The model under review builds one solid part; all positions refer to its coordinate system, in mm. A direction names the side the tool comes from. Round coordinates to 2 decimals unless told otherwise and drop trailing zeros. Write each loop counter-clockwise with the first axis right and the second up, starting at its lowest first coordinate (ties: lowest second). Pieces come first, ordered by that corner, then holes. Notation, with made-up numbers: (65, 50) -> (84, 50) arc R22 cw to (84, 68) -> close; hole circle Ø5 at (-35, 16.25). An arc over 180 degrees is marked (long way). Return JSON: item names as keys, results as strings. Group by question number.
1. Take a section at D-D, the plane x = 2.5. Write out the cut boundary in (y, z), then the cut area to 3 significant figures.
2. Clearance check with flat-ended pins moving along their axes: P1, Ø4, axis at y = 3.5, z = -2.5, coming from the -X side; P2, Ø3, axis at x = -40, y = 3.5, coming from the -Z side; P3, Ø4, axis at x = -3.5, y = 2, coming from the +Z side. State where each tip first meets the part, or that it passes through.
3. Take a section at A-A, the plane z = -2.5. Write out the cut boundary in (x, y).
4. For line 1 along Y through (x, z) = (4.5, -2.5); line 2 along X through (y, z) = (3.5, 9.75); line 3 along X through (y, z) = (3.5, 12.75), list the stretches that pass through material, from the lowest coordinate up. Write a range as from..to.
5. Tool access review of faces 1 (the flat face through (-22, 3, 7.5)), 2 (the flat face through (7, 3, -18)), 3 (the flat face through (-27, 3, 14.5)), 4 (the flat face through (3, 3, -35)): name each direction out of +Z, -Z, +X, -X, +Y, -Y from which nothing blocks a thin tool from reaching the whole face with its end or side.
6. Take a section at B-B, the plane x = -10. Write out the cut boundary in (y, z), then the cut area to 3 significant figures.
7. Mouldability with a two-part tool opening along Z and no side actions: class faces 5 (the flat face through (2.59, 3.45, 20.65)), 6 (the cylindrical face through (-39.01, 2.74, 10.95)), 7 (the cylindrical face through (3.451, 3.021, -31.345)) as pulls with the +Z half, pulls with the -Z half, needs draft (parallel to the pull), parting line crosses it, or undercut.
8. Take a section at C-C, the plane y = 1. Write out the cut boundary in (x, z).
Autodesk Inventor part; units mm, degrees
ref_plane "YZ Plane" through (0, 0, 0) normal (1, 0, 0) x (0, 1, 0)
ref_plane "XZ Plane" through (0, 0, 0) normal (0, 1, 0) x (-1, 0, 0)
ref_plane "XY Plane" through (0, 0, 0) normal (0, 0, 1) x (1, 0, 0)
sketch "Sketch1" plane through (0, 0, 0) normal (0, 1, 0) x (-1, 0, 0)
  line L0 (0, 0) -> (16.4443, 0)
  line L1 (0, 0) -> (0, -35)
  line L2 (0, -17.5) -> (0, 7.5)
  line L3 (0, 7.5) -> (45, 7.5)
  line L4 (0, -35) -> (-7, -35)
  line L5 (-7, -35) -> (-7, 14.5)
  line L6 (8.8556, 14.5) -> (45, 14.5)
  line L7 (45, 14.5) -> (45, 7.5)
  line L8 (0, 7.5) -> (-14.2941, 21.7941)
  line L9 (0, 7.5) -> (20.2149, 7.5) construction
  circle A0 centre (-14.2941, 21.7941) radius 3
  circle A1 centre (-14.2941, 21.7941) radius 5
  line L10 (-11.7387, 26.0918) -> (6.8113, 15.0619)
  arc A2 (6.8113, 15.0619) -> (8.8556, 14.5) centre (8.8556, 18.5) ccw
  line L11 (-18.5918, 19.2387) -> (-7.5619, 0.6887)
  arc A3 (-7, -1.3556) -> (-7.5619, 0.6887) centre (-11, -1.3556) ccw
  point P0 (-7, -1.3556)
  dimension "d8" = 10
  dimension "d0" = 35
  dimension "d2" = 25
  dimension "d3" = 45
  dimension "d4" = 7
  dimension "d5" = 7
  dimension "d6" = 135
  dimension "d7" = 6
  dimension "d9" = 4
extrude "Extrusion1" add sketch "Sketch1" along normal blind 7
sketch "Sketch2" plane through (0, 0, -35) normal (-1, 0, 0) x (0, 0, 1)
  line L0 (42.5, 0) -> (42.5, 7)
  line L1 (42.5, 3.5) -> (32.5, 3.5)
  line L2 (32.5, 3.5) -> (2.5, 3.5)
  circle A0 centre (32.5, 3.5) radius 1.25
  circle A1 centre (2.5, 3.5) radius 1.25
  point P0 (35, 0)
  dimension "d12" = 10
  dimension "d13" = 30
  dimension "d14" = 2.5
  dimension "d15" = 2.5
extrude "Extrusion2" cut sketch "Sketch2" against normal through all
sketch "Sketch3" plane through (0, 0, 7.5) normal (0, 0, -1) x (-1, 0, 0)
  line L0 (0, 0) -> (0, 7)
  line L1 (0, 3.5) -> (10, 3.5)
  line L2 (10, 3.5) -> (40, 3.5)
  circle A0 centre (40, 3.5) radius 1.25
  circle A1 centre (10, 3.5) radius 1.25
  dimension "d18" = 10
  dimension "d19" = 30
  dimension "d20" = 2.5
  dimension "d21" = 2.5
extrude "Extrusion3" cut sketch "Sketch3" against normal blind 10
properties part number "GPSholder" material "PC/ABS Plastic"
Output:
{
 "1": {"outline": "(0, -35) -> (7, -35) -> (7, 20.6) -> (0, 20.6) -> close; hole circle Ø2.5 at (3.5, -32.5); hole circle Ø2.5 at (3.5, -2.5)", "area": "379 mm^2"},
 "2": {"P1": "stops at x = 0", "P2": "stops at z = 7.5", "P3": "stops at z = 18.22"},
 "3": {"outline": "(0, 0) -> (7, 0) -> (7, 2.25) -> (0, 2.25) -> close; (0, 4.75) -> (7, 4.75) -> (7, 7) -> (0, 7) -> close"},
 "4": {"line 1": "y = 0..2.25, 4.75..7", "line 2": "x = -45..-41.25, -38.75..-11.25, -8.75..12.95", "line 3": "x = -45..-41.25, -38.75..-11.25, -8.75..14.73"},
 "5": {"face 1": "-Z, -X, +Y, -Y", "face 2": "-Z, +X, +Y, -Y", "face 3": "+Z, -X, +Y, -Y", "face 4": "-Z, +X, -X, +Y, -Y"},
 "6": {"outline": "(0, 7.5) -> (2.25, 7.5) -> (2.25, 14.5) -> (0, 14.5) -> close; (4.75, 7.5) -> (7, 7.5) -> (7, 14.5) -> (4.75, 14.5) -> close", "area": "31.5 mm^2"},
 "7": {"face 5": "pulls with the +Z half", "face 6": "needs draft", "face 7": "undercut"},
 "8": {"outline": "(-45, 7.5) -> (0, 7.5) -> (0, -35) -> (7, -35) -> (7, -1.36) arc R4 cw to (7.56, 0.69) -> (18.59, 19.24) arc R5 ccw to (11.74, 26.09) -> (-6.81, 15.06) arc R4 cw to (-8.86, 14.5) -> (-45, 14.5) -> close; hole circle Ø6 at (14.29, 21.79)"}
}
